Autodesk Inventor part; units mm, degrees
ref_plane "YZ Plane" through (0, 0, 0) normal (1, 0, 0) x (0, 1, 0)
ref_plane "XZ Plane" through (0, 0, 0) normal (0, 1, 0) x (-1, 0, 0)
ref_plane "XY Plane" through (0, 0, 0) normal (0, 0, 1) x (1, 0, 0)
sketch "Sketch1" plane through (0, 0, 0) normal (0, 1, 0) x (-1, 0, 0)
  circle A0 centre (0, 0) radius 8
  dimension "d0" = 16
extrude "Extrusion1" add sketch "Sketch1" along normal blind 2
sketch "Sketch2" plane through (0, 2, 0) normal (0, 1, 0) x (1, 0, 0)
  circle A0 centre (0, 0) radius 8
  circle A1 centre (0, 0) radius 6.1
  dimension "d3" = 12.2
extrude "Extrusion2" add sketch "Sketch2" along normal blind 7 contours A1
sketch "Sketch3" plane through (0, 9, 0) normal (0, 1, 0) x (1, 0, 0)
  circle A0 centre (0, 0) radius 6.1
  circle A1 centre (0, 0) radius 8
extrude "Extrusion3" add sketch "Sketch3" along normal blind 7 contours A0 | A1
sketch "Sketch4" plane through (0, 16, 0) normal (0, 1, 0) x (1, 0, 0)
  circle A0 centre (0, 0) radius 2.5
  dimension "d8" = 5
extrude "Extrusion4" cut sketch "Sketch4" against normal through all
properties part number "GT2_5mm_Pulley"
The model under review builds one solid part; all positions refer to its coordinate system, in mm. A direction names the side the tool comes from. Round coordinates to 2 decimals unless told otherwise and drop trailing zeros. Order: outer loops, then holes, each group sorted by start corner. A loop starts at its lowest first (then second) coordinate and runs counter-clockwise, first axis right, second up.
(1) Tool access review of faces 1 (the face through (2, 0, -2)), 2 (the face through (-6.094, 5.451, 0.268)): name each direction out of +Z, -Z, +X, -X, +Y, -Y from which nothing blocks a thin tool from reaching the whole face with its end or side.
Working result:
face 1: +Z, -Z, +X, -X, -Y
face 2: none
(2) Take a section at C-C, the plane y = 11.25. State the section outline as (x, z) points, plus the area to 3 significant figures.
Working result:
outline: circle Ø16 at (0, 0); hole circle Ø5 at (0, 0)
area: 181 mm2
(3) Take a section at A-A, the plane z = 0. State the section outline as (x, y) points, plus the area to 3 significant figures.
Working result:
outline: (-8, 0) - (-2.5, 0) - (-2.5, 16) - (-8, 16) - (-8, 9) - (-6.1, 9) - (-6.1, 2) - (-8, 2) - close; (2.5, 0) - (8, 0) - (8, 2) - (6.1, 2) - (6.1, 9) - (8, 9) - (8, 16) - (2.5, 16) - close
area: 149 mm2
(4) Mouldability with a two-part tool opening along Y and no side actions: class faces 3 (the face through (-0.54, 8.11, 2.44)), 4 (the face through (-2, 9, 6)), 5 (the face through (-2, 16, 2)) as released by +Y, released by -Y, zero draft, split by the parting line, or undercut.
Working result:
face 3: zero draft
face 4: undercut
face 5: released by +Y
(5) For P1, Ø4, axis at y = 7.5, z = -1, coming from the -X side; P2, Ø1.5, axis at x = 3, y = 4.5, coming from the -Z side; P3, Ø2, axis at x = 2, y = 8.5, coming from the +Z side, all flat-tipped, find the tip position at first contact; note any pin that passes through.
Working result:
P1: stops at x = -8
P2: stops at z = -5.67
P3: stops at z = 7.92
(6) Take a section at B-B, the plane x = 0. State the section outline as (y, z) points, plus the area to 3 significant figures.
Working result:
outline: (0, -8) - (2, -8) - (2, -6.1) - (9, -6.1) - (9, -8) - (16, -8) - (16, -2.5) - (0, -2.5) - close; (0, 2.5) - (16, 2.5) - (16, 8) - (9, 8) - (9, 6.1) - (2, 6.1) - (2, 8) - (0, 8) - close
area: 149 mm2
(7) Take a section at D-D, the plane x = 5. State the section outline as (y, z) points (3 decimals), plus the area to 3 significant figures.
Working result:
outline: (0, -6.245) - (2, -6.245) - (2, -3.494) - (9, -3.494) - (9, -6.245) - (16, -6.245) - (16, 6.245) - (9, 6.245) - (9, 3.494) - (2, 3.494) - (2, 6.245) - (0, 6.245) - close
area: 161 mm2
(8) Wall thickness on L1, parallel to Z at x = 0, y = 10; L2, parallel to Z at x = 0, y = 8.5: over which ranges is each line inside the solid? List them lowest first.
Working result:
L1: z = -8 to -2.5, 2.5 to 8
L2: z = -6.1 to -2.5, 2.5 to 6.1
